Could you check a few things on this model? Use its own coordinates, in mm. A direction names the side the tool comes from. Coordinates: 2 decimals unless noted, no trailing zeros. Order: outer loops, then holes, each group sorted by start corner. A loop starts at its lowest first (then second) coordinate and runs counter-clockwise, first axis right, second up. Notation, with made-up numbers: (-35, 63) -> (-9, 63) arc R11 cw to (-9, 68) -> close; hole circle Ø8 at (-34.5, 38.25). An arc over 180 degrees is marked (long way). Put each result on its own line as item: value. Start each with the question number.
Q1. We'd pull the mould along X, two halves only. Please class faces 5 (the face through (0, 22, 0)), 6 (the face through (7.91, 18.056, -10.316)), 7 (the face through (7.784, 19.972, 1.115)): +X half, -X half, draft (parallel to the pull), parting line (faces both ways), or undercut.
Q2. If we section it at A-A (y = 14.5): Please give me the cut outline in (x, z).
Q3. For faces 1 (the face through (-10.65, 19.97, 0.07)), 2 (the face through (3.905, 13.014, -0.867)), 3 (the face through (0, 0, 0)), 4 (the face through (0, 7, -5)), which set-ups out of +Z, -Z, +X, -X, +Y, -Y let a thin tool reach every point of the face, with its end or its side?
Q4. If we section it at B-B (z = 8.5): Please give me the cut outline in (x, y).
Q5. Please list where these lines run through material, in increasing order: line 1 along X through (y, z) = (19.3, 0); line 2 along Z through (x, y) = (9.75, 19.5); line 3 along Z through (x, y) = (9, 21.15).
Q6. If we section it at C-C (y = 4.5): Please give me the cut outline in (x, z), and give its area (3 significant figures).
Q7. Will these pins go through, and if not, where does the flat tip stop? pin 1 (8 mm diameter, centred on x = -4, z = -8.5, fed in from -Y); pin 2 (6 mm diameter, centred on x = -3.5, z = 3, fed in from -Y); pin 3 (1.5 mm diameter, centred on y = 14, z = 2, fed in from +X); pin 4 (2 mm diameter, centred on x = -4.5, y = 9, fed in from -Z).
Q8. If we section it at D-D (x = -6): Please give me the cut outline in (y, z), and give its area (3 significant figures).
from build123d import *

# Parameters (mm, degrees)
CHAMFER_1_SIZE         = 2
HOLE_WIZARD_M4_1_D     = 3.3
HOLE_WIZARD_M4_1_DEPTH = 4
HOLE_WIZARD_M4_1_TIP   = 0.991420021


with BuildPart() as part:
    # 草图1 → 旋转1 (revolve)
    with BuildSketch(Plane.XY, mode=Mode.PRIVATE) as revolve_1_sk:
        Polygon((0, 0), (5, 0), (5, 12), (4, 12), (4, 14), (13, 14), (13, 22), (0, 22), align=None)
    revolve(revolve_1_sk.sketch.rotate(Axis((0, 60.790955631, 0), (0, -1, 0)), 90), axis=Axis((0, 60.790955631, 0), (0, -1, 0)))

    # 倒角1
    chamfer_1_edges = [part.edges().sort_by_distance(p)[0] for p in [
        (0, 0, -5),
    ]]
    chamfer(chamfer_1_edges, length=CHAMFER_1_SIZE)

    # M4 螺纹孔的螺纹孔钻头1
    with Locations(Plane(origin=(0, 22, 0), x_dir=(-1, 0, 0), z_dir=(0, 1, 0))):
        with Locations((9, 0), (-9, 0)):
            Hole(HOLE_WIZARD_M4_1_D / 2, depth=HOLE_WIZARD_M4_1_DEPTH)
            with Locations((0, 0, -(HOLE_WIZARD_M4_1_DEPTH + HOLE_WIZARD_M4_1_TIP / 2))):  # 118° drill point
                Cone(0, HOLE_WIZARD_M4_1_D / 2, HOLE_WIZARD_M4_1_TIP, mode=Mode.SUBTRACT)


solid = part.part
The answers:
1. face 5: draft
1. face 6: parting line
1. face 7: undercut
2. outline: circle Ø26 at (0, 0)
3. face 1: +Y
3. face 2: none
3. face 3: +Z, -Z, +X, -X, -Y
3. face 4: -Y
4. outline: (-9.84, 14) -> (9.84, 14) -> (9.84, 22) -> (-9.84, 22) -> close
5. line 1: -13 to -10.65, -7.35 to 7.35, 10.65 to 13
5. line 2: -8.6 to -1.47, 1.47 to 8.6
5. line 3: -9.38 to -1.65, 1.65 to 9.38
6. outline: circle Ø10 at (0, 0)
6. area: 78.5 mm^2
7. pin 1: y = 14
7. pin 2: y = 0
7. pin 3: x = 12.94
7. pin 4: z = -3.57
8. outline: (14, -11.53) -> (22, -11.53) -> (22, 11.53) -> (14, 11.53) -> close
8. area: 185 mm^2
